Design review of the part built by this model. Coordinates are the model's own, in mm. A direction names the side the tool comes from. Coordinates: 2 decimals unless noted, no trailing zeros. Loops run counter-clockwise (first coordinate to the right, second up) from the corner with the lowest first, then second, coordinate; pieces in that order, holes last. Notation, with made-up numbers: (39.25, 48) -> (57.25, 48) arc R19 cw to (57.25, 82) -> close; hole circle Ø3 at (55.25, 71). An arc over 180 degrees is marked (long way). Use one line per item in the form item = value. Start each with the question number.
1. The part is to be moulded in two halves that separate along X. For faces 5 (the face through (-4.167, 0.133, 11.98)), 6 (the face through (-38.097, 0.391, 32.088)), 7 (the face through (-1, 9, 1.588)), say which applies: released by +X, released by -X, zero draft, split by the parting line, or undercut.
2. Wall thickness on line 1 (Z direction, x = 0, y = 5); line 2 (Z direction, x = 30, y = -13); line 3 (X direction, y = 0, z = 38.5): over which ranges is each line inside the solid? List them lowest first. Write a range as from..to.
3. Machinability: for faces 1 (the face through (-1, -9, 1.588)), 2 (the face through (-1, 0, 0)), 3 (the face through (-15.875, -16, 16)), 4 (the face through (0, 16, 31.75)), which of the approach directions +Z, -Z, +X, -X, +Y, -Y give a long, thin tool a straight path to every point of the face, cutting with its end or side? Answer none if there is none.
4. For pin 1 (1 mm diameter, centred on x = 9.5, z = 21, fed in from +Y) (3 decimals); pin 2 (2.5 mm diameter, centred on x = -11.5, y = 9.5, fed in from -Z); pin 3 (4 mm diameter, centred on x = 1, y = -14, fed in from -Z), all flat-tipped, find the tip position at first contact; note any pin that passes through.
5. Consider section D-D (z = 55). State the section outline as (x, y) points (1 decimal), then the cut area to 3 significant figures.
6. Consider section C-C (z = 28). State the section outline as (x, y) points (1 decimal), then the cut area to 3 significant figures.
from build123d import *

# Parameters (mm, degrees)
F1_DEPTH = 65.0875
F2_W     = 31.75
F2_H     = 8.73125
F3_DEPTH = 31.75
F4_DEPTH = 1.5875
F6_D     = 8.7376


with BuildPart() as f1:
    # F0 (on Top) → F1 (new body)
    with BuildSketch(Plane.XY):
        with BuildLine():
            ThreePointArc((-23.8125, 22.225), (-38.1, 0), (-23.8125, -22.225))
            Line((-23.8125, -22.225), (23.8125, -22.225))
            ThreePointArc((23.8125, -22.225), (38.1, 0), (23.8125, 22.225))
            Line((23.8125, 22.225), (-23.8125, 22.225))
        make_face()
    extrude(amount=F1_DEPTH)

    # F2 (on face) → F3 (cut)
    with BuildSketch(Plane(origin=(0, 0, 0), x_dir=(1, 0, 0), z_dir=(0, 0, -1))):
        with Locations((0, 17.859375)):
            Rectangle(F2_W, F2_H)
        Polygon((15.875, 13.49375), (-15.875, 13.49375), (-15.875, 9.525), (0, 9.525), (15.875, 9.525), align=None)
        with Locations((0, -17.859375)):
            Rectangle(F2_W, F2_H)
        Polygon((-15.875, -9.525), (-15.875, -13.49375), (15.875, -13.49375), (15.875, -9.525), (0, -9.525), align=None)
    extrude(amount=-F3_DEPTH, mode=Mode.SUBTRACT)

    # F2 (on face) → F4 (cut)
    with BuildSketch(Plane(origin=(0, 0, 0), x_dir=(1, 0, 0), z_dir=(0, 0, -1))):
        with BuildLine():
            Line((-15.875, 13.49375), (-34.0352272718, 13.49375))
            ThreePointArc((-34.0352272718, 13.49375), (-36.1013811244, 9.6776797674), (-37.4597626742, 5.55625))
            Line((-37.4597626742, 5.55625), (37.4597626742, 5.55625))
            ThreePointArc((37.4597626742, 5.55625), (36.1013811244, 9.6776797674), (34.0352272718, 13.49375))
            Line((34.0352272718, 13.49375), (15.875, 13.49375))
            Line((15.875, 13.49375), (15.875, 9.525))
            Line((15.875, 9.525), (0, 9.525))
            Line((0, 9.525), (-15.875, 9.525))
            Line((-15.875, 9.525), (-15.875, 13.49375))
        make_face()
        with BuildLine():
            Line((37.4597626742, -5.55625), (-37.4597626742, -5.55625))
            ThreePointArc((-37.4597626742, -5.55625), (-36.1013811244, -9.6776797674), (-34.0352272718, -13.49375))
            Line((-34.0352272718, -13.49375), (-15.875, -13.49375))
            Line((-15.875, -13.49375), (-15.875, -9.525))
            Line((-15.875, -9.525), (0, -9.525))
            Line((0, -9.525), (15.875, -9.525))
            Line((15.875, -9.525), (15.875, -13.49375))
            Line((15.875, -13.49375), (34.0352272718, -13.49375))
            ThreePointArc((34.0352272718, -13.49375), (36.1013811244, -9.6776797674), (37.4597626742, -5.55625))
        make_face()
    extrude(amount=-F4_DEPTH, mode=Mode.SUBTRACT)

    # F6 (through all)
    with Locations(Plane.XZ.offset(9.525)):
        with Locations((0, 10.668)):
            Hole(F6_D / 2)


solid = f1.part
Geometry check:
q1.face_5 = undercut
q1.face_6 = released by -X
q1.face_7 = zero draft
q2.line_1 = 0..6.3, 15.04..65.09
q2.line_2 = 1.59..65.09
q2.line_3 = -38.1..38.1
q3.face_1 = -Z, +X, -X
q3.face_2 = -Z, +X, -X, +Y, -Y
q3.face_3 = -Z, -Y
q3.face_4 = -Z, +Y
q4.pin_1 = 9.525
q4.pin_2 = 1.59
q4.pin_3 = 31.75
q5.outline = (-23.8, -22.2) -> (23.8, -22.2) arc R24.4 ccw to (23.8, 22.2) -> (-23.8, 22.2) arc R24.4 ccw to start
q5.area = 3,030 mm²
q6.outline = (-23.8, -22.2) -> (-15.9, -22.2) -> (-15.9, -9.5) -> (15.9, -9.5) -> (15.9, -22.2) -> (23.8, -22.2) arc R24.4 ccw to (23.8, 22.2) -> (15.9, 22.2) -> (15.9, 9.5) -> (-15.9, 9.5) -> (-15.9, 22.2) -> (-23.8, 22.2) arc R24.4 ccw to start
q6.area = 2,220 mm²
